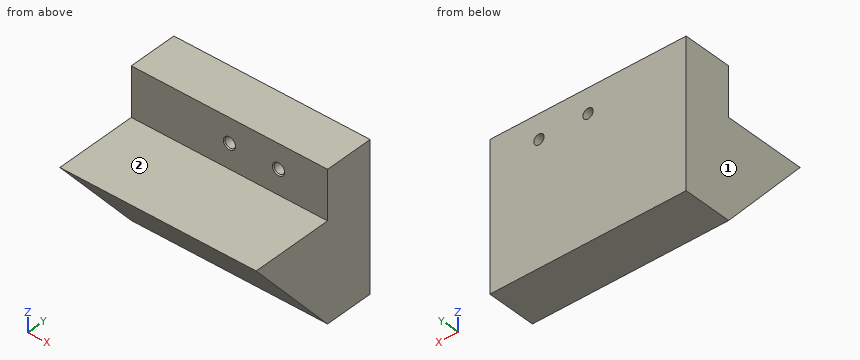
Solid Edge part; units mm, degrees
sketch "Sketch1" plane through (0, 0, 0) normal (0, -1, 0) x (1, 0, 0)
  line L0 (0, 0) -> (200, 0)
  line L1 (200, 0) -> (200, 150)
  line L2 (200, 150) -> (0, 150)
  line L3 (0, 150) -> (0, 0)
extrude "Protrusion1" add sketch "Sketch1" against normal blind 50
sketch "Sketch2" plane through (0, 25, 75) normal (-1, 0, 0) x (0, 0, -1)
  line L0 (75, 25) -> (-25, 108.91)
  line L1 (-25, 108.91) -> (-25, 25)
  line L2 (-25, 25) -> (75, 25)
extrude "Extrusionsausprägung_2" add sketch "Sketch2" against normal blind 200
hole "Bohrung_1" at (100, 0, 125) direction (0, 1, 0) diameter 10.5 end up to next start chamfer 1 start chamfer angle 45
hole "Hole1" at (150, 0, 125) direction (0, 1, 0) diameter 10.5 end up to next start chamfer 1 start chamfer angle 45
Source: CAD feature listing. Evaluate the final solid. Frame: model axes, mm. Face numbers are marked on the shaded views. A direction names the side the tool comes from. Give positions to 0.01 mm unless a question says otherwise; leave off trailing zeros. Loops run counter-clockwise (first coordinate to the right, second up) from the corner with the lowest first, then second, coordinate; pieces in that order, holes last. Notation, with made-up numbers: M -12.75,66 L 5.25,66 A13 ccw 5.25,72 Z; hole C -18.5,78.5 d5. An arc over 180 degrees is marked long. Put each result on its own line as item: value.
Q1. Section C-C (x = 74). Return the cut outline in (y, z).
Response values:
outline: M -83.91,100 L 0,0 L 50,0 L 50,150 L 0,150 L 0,100 Z
Q2. Pin query (flat end, axial travel): P1, Ø1.5, axis at x = 97, z = 78.5, coming from the -Y side; P2, Ø5, axis at x = 155.5, z = 82, coming from the -Y side; P3, Ø8.5, axis at x = 100, z = 125, coming from the -Y side; P4, Ø8, axis at x = 68.5, z = 126, coming from the -Y side. Return the tip coordinate at first contact, or that it passes through.
Response values:
P1: stops at y = -66.5
P2: stops at y = -70.9
P3: passes through
P4: stops at y = 0
Q3. Line query: probe 1 along X at (y, z) = (24.5, 125); probe 2 along Z at (x, y) = (100, 19); probe 3 along Y at (x, z) = (111, 128.5). Output: solid intervals per line, ascending. Write a range as [from, to].
Response values:
probe 1: x = [0, 94.75], [105.25, 144.75], [155.25, 200]
probe 2: z = [0, 119.75], [130.25, 150]
probe 3: y = [0, 50]
Q4. Section B-B (x = 100). Return the cut outline in (y, z), and give its area (3 significant figures).
Response values:
outline: M -83.91,100 L 0,0 L 50,0 L 50,119.75 L 1,119.75 L 0,118.75 L 0,100 Z; M 0,131.25 L 1,130.25 L 50,130.25 L 50,150 L 0,150 Z
area: 11,200 mm²
Q5. Reachability of the marked faces 1 and 2 from +Z, -Z, +X, -X, +Y, -Y: full face, straight path, thin tool, end or side. Return the list, or none.
Response values:
face 1: +Z, -Z, -X, +Y, -Y
face 2: +Z, +X, -X, -Y
Q6. Section A-A (z = 125). Return the cut outline in (x, y), and give its area (3 significant figures).
Response values:
outline: M 0,0 L 93.75,0 L 94.75,1 L 94.75,50 L 0,50 Z; M 105.25,1 L 106.25,0 L 143.75,0 L 144.75,1 L 144.75,50 L 105.25,50 Z; M 155.25,1 L 156.25,0 L 200,0 L 200,50 L 155.25,50 Z
area: 8,950 mm²
Q7. Section D-D (z = 60). Return the cut outline in (x, y).
Response values:
outline: M 0,-50.35 L 200,-50.35 L 200,50 L 0,50 Z
